Geometry: final body of the model. Coordinates: model frame, mm. A direction names the side the tool comes from. Round coordinates to 2 decimals unless told otherwise and drop trailing zeros. Loops run counter-clockwise (first coordinate to the right, second up) from the corner with the lowest first, then second, coordinate; pieces in that order, holes last. Notation, with made-up numbers: M 31.5,63.5 L 63.5,63.5 A16 cw 63.5,83.5 Z; hole C 17,71.5 d9. An arc over 180 degrees is marked long. Answer as a JSON object with one key per item and string values.
from build123d import *

# Parameters (mm, degrees)
HEX_START                = 11.30066774
HEX_OUTER_SIDE_OUTLINE_W = 3.302
HEX_OUTER_SIDE_OUTLINE_H = 7.747
HEX_OUTER_SIDE_OUTLINE_R = 1.5875
HEX_OUTER_SIDE_DEPTH     = 3.175
SKETCH1_R                = 3.4925
CUT_EXTRUDE1_DEPTH       = 3.175


# Read off the part's stored shape, not the designer's step: Hex Outer Side
with BuildPart() as part:
    # Hex Outer Side outline → Hex Outer Side (new body)
    with BuildSketch(Plane(origin=(0, 0, 0), x_dir=(1, 0, 0), z_dir=(0, 1, 0)).offset(HEX_START)):
        with BuildLine():
            Line((-47.528050259, 17.731483109), (-47.528050259, -1.318516891))
            ThreePointArc((-47.528050259, -1.318516891), (-45.66817832, -5.808644951), (-41.178050259, -7.668516891))
            Line((-41.178050259, -7.668516891), (10.256949741, -7.668516891))
            Line((10.256949741, -7.668516891), (10.256949741, -5.128516891))
            Line((10.256949741, -5.128516891), (13.431949741, -5.128516891))
            Line((13.431949741, -5.128516891), (13.431949741, 2.491483109))
            Line((13.431949741, 2.491483109), (10.256949741, 2.491483109))
            Line((10.256949741, 2.491483109), (10.256949741, 5.031483109))
            Line((10.256949741, 5.031483109), (-34.828050259, 5.031483109))
            Line((-34.828050259, 5.031483109), (-34.828050259, 17.731483109))
            ThreePointArc((-34.828050259, 17.731483109), (-36.687922199, 22.22161117), (-41.178050259, 24.081483109))
            ThreePointArc((-41.178050259, 24.081483109), (-45.668178319, 22.221611169), (-47.528050259, 17.731483109))
        make_face()
        with Locations((-26.954050259, -1.318516891)):
            Rectangle(HEX_OUTER_SIDE_OUTLINE_W, HEX_OUTER_SIDE_OUTLINE_H, mode=Mode.SUBTRACT)
        with Locations((-41.178050259, 20.906483109)):
            Circle(HEX_OUTER_SIDE_OUTLINE_R, mode=Mode.SUBTRACT)
    extrude(amount=HEX_OUTER_SIDE_DEPTH)

    # Sketch1 → Cut-Extrude1 (cut)
    with BuildSketch(Plane(origin=(0, 14.47566774, 0), x_dir=(1, 0, 0), z_dir=(0, 1, 0))):
        with Locations(Location((-7.523050259, -1.318516891, 0), (0, 0, 270))):
            Circle(SKETCH1_R)
    extrude(amount=-CUT_EXTRUDE1_DEPTH, mode=Mode.SUBTRACT)


solid = part.part
1) Pull-direction query (X, two-part tool) for faces 1 (the flat face through (-24, 14.476, -1)), 2 (the cylindrical face through (-10.62, 12.91, 2.93)), 3 (the flat face through (-27, 13, 5.192)), 4 (the flat face through (10.257, 13, -4)); classes: +X half, -X half, draft (parallel to the pull), parting line (faces both ways), or undercut.
Results:
{"face 1": "draft", "face 2": "undercut", "face 3": "undercut", "face 4": "+X half"}
2) Pin query (flat end, axial travel): P1, Ø1.5, axis at x = -8.5, y = 13, coming from the -Z side; P2, Ø1, axis at y = 13.5, z = -9.5, coming from the +X side; P3, Ø1.3, axis at y = 13, z = 7, coming from the +X side. Return the tip coordinate at first contact, or that it passes through.
Results:
{"P1": "z = -5.03", "P2": "x = -34.83", "P3": "x = 10.26"}
3) Ray query, line 1 (X direction, y = 13.45, z = 2); line 2 (X direction, y = 14.15, z = 4); line 3 (X direction, y = 12.3, z = -16.5). Return the intervals inside material, ascending.
Results:
{"line 1": "-47.49 to -28.61, -25.3 to -10.95, -4.1 to 13.43", "line 2": "-46.93 to -28.61, -25.3 to -9.76, -5.29 to 13.43", "line 3": "-47.53 to -34.83"}
4) Section query D-D (z = -17). Return the cut outline in (x, y), and give its area (3 significant figures).
Results:
{"outline": "M -47.53,11.3 L -34.83,11.3 L -34.83,14.48 L -47.53,14.48 Z", "area": "40.3 mm2"}
5) Section query A-A (z = 3.5). Return the cut outline in (x, y).
Results:
{"outline": "M -47.14,11.3 L -28.61,11.3 L -28.61,14.48 L -47.14,14.48 Z; M -25.3,11.3 L -10.25,11.3 L -10.25,14.48 L -25.3,14.48 Z; M -4.8,11.3 L 13.43,11.3 L 13.43,14.48 L -4.8,14.48 Z"}
6) Section query B-B (x = -6.5). Return the cut outline in (y, z).
Results:
{"outline": "M 11.3,-5.03 L 14.48,-5.03 L 14.48,-2.02 L 11.3,-2.02 Z; M 11.3,4.66 L 14.48,4.66 L 14.48,7.67 L 11.3,7.67 Z"}
7) Reachability of faces 5 (the flat face through (-16, 13, 7.669)), 6 (the flat face through (13.432, 13, 1)), 7 (the flat face through (-12, 13, -5.031)), 8 (the flat face through (12, 13, 5.129)), 9 (the flat face through (-28.605, 13, 1)) from +Z, -Z, +X, -X, +Y, -Y: full face, straight path, thin tool, end or side. Return the list, or none.
Results:
{"face 5": "+Z, +X, -X, +Y, -Y", "face 6": "+Z, -Z, +X, +Y, -Y", "face 7": "-Z, +X, +Y, -Y", "face 8": "+Z, +X, +Y, -Y", "face 9": "+Y, -Y"}
8) Section query C-C (y = 13.25). Count the separate pieces of the cut face and the enclosed holes in it, and give its area (3 significant figures).
Results:
{"separate pieces": "1", "enclosed holes": "3", "area": "902 mm2"}
